from build123d import *

# Parameters (mm, degrees)
BOSS_EXTRUDE2_DEPTH = 100
SKETCH3_W           = 90
SKETCH3_H           = 32.5
CUT_EXTRUDE1_DEPTH  = 60


with BuildPart() as part:
    # Sketch2 → Boss-Extrude2 (new body)
    with BuildSketch(Plane(origin=(0, 0, 0), x_dir=(0, 0, -1), z_dir=(1, 0, 0))):
        Polygon((42.5, 60), (0, 17.5), (0, 0), (42.5, 0), align=None)
    extrude(amount=BOSS_EXTRUDE2_DEPTH)

    # Sketch3 → Cut-Extrude1 (cut)
    with BuildSketch(Plane.XZ):
        with Locations((50, -21.25)):
            Rectangle(SKETCH3_W, SKETCH3_H)
    extrude(amount=-CUT_EXTRUDE1_DEPTH, mode=Mode.SUBTRACT)


solid = part.part
Input: part model. Units: mm. Frame: model coordinates. A direction names the side the tool comes from. Give positions to 0.01 mm unless a question says otherwise; leave off trailing zeros. Loops run counter-clockwise (first coordinate to the right, second up) from the corner with the lowest first, then second, coordinate; pieces in that order, holes last. Notation, with made-up numbers: (23, 56.25) -> (52, 56.25) arc R35 cw to (52, 91.25) -> close; hole circle Ø6 at (2.5, 0.5). An arc over 180 degrees is marked (long way). Answer as a JSON object with one key per item and string values. Group by question number.
Item 1: Line query: probe 1 along Z at (x, y) = (25.5, 4.5); probe 2 along X at (y, z) = (16.5, -28.5); probe 3 along Z at (x, y) = (56, 52). Output: solid intervals per line, ascending.
Item 2: Cut plane D-D, the plane y = 48. Return the cut outline in (x, z), and give its area (3 significant figures).
Item 3: Reachability of faces 1 (the flat face through (46, 0, -4)), 2 (the flat face through (95, 21, -25)) from +Z, -Z, +X, -X, +Y, -Y: full face, straight path, thin tool, end or side. Return the list, or none.
Item 4: Cut plane A-A, the plane z = -31. Return the cut outline in (x, y), and give its area (3 significant figures).
Item 5: Pin query (flat end, axial travel): P1, Ø6, axis at x = 15.5, y = 37.5, coming from the +Z side. Return the tip coordinate at first contact, or that it passes through.
Item 6: Cut plane C-C, the plane y = 20.5. Return the cut outline in (x, z), and give its area (4 significant figures).
Item 7: Pull-direction query (X, two-part tool) for faces 3 (the flat face through (49, 11, -5)), 4 (the flat face through (49, 30, -42.5)), 5 (the flat face through (0, 24, -26)), 6 (the flat face through (49, 27, -37.5)); classes: released by +X, released by -X, zero draft, split by the parting line, or undercut.
Item 8: Cut plane B-B, the plane x = 47. Return the cut outline in (y, z), and give its area (4 significant figures).
Checks:
{
 "1": {"probe 1": "z = -42.5 to -37.5, -5 to 0", "probe 2": "x = 0 to 5, 95 to 100", "probe 3": "z = -42.5 to -37.5"},
 "2": {"outline": "(0, -42.5) -> (100, -42.5) -> (100, -30.5) -> (95, -30.5) -> (95, -37.5) -> (5, -37.5) -> (5, -30.5) -> (0, -30.5) -> close", "area": "570 mm²"},
 "3": {"face 1": "+Z, -Z, +X, -X, -Y", "face 2": "+Y, -Y"},
 "4": {"outline": "(0, 0) -> (5, 0) -> (5, 48.5) -> (0, 48.5) -> close; (95, 0) -> (100, 0) -> (100, 48.5) -> (95, 48.5) -> close", "area": "485 mm²"},
 "5": {"P1": "stops at z = -37.5"},
 "6": {"outline": "(0, -42.5) -> (100, -42.5) -> (100, -3) -> (0, -3) -> close; hole (5, -37.5) -> (95, -37.5) -> (95, -5) -> (5, -5) -> close", "area": "1,025 mm²"},
 "7": {"face 3": "undercut", "face 4": "zero draft", "face 5": "released by -X", "face 6": "undercut"},
 "8": {"outline": "(0, -42.5) -> (60, -42.5) -> (55, -37.5) -> (0, -37.5) -> close; (0, -5) -> (22.5, -5) -> (17.5, 0) -> (0, 0) -> close", "area": "387.5 mm²"}
}
